Geometry: final body of the model. Coordinates: model frame, mm. Face numbers are marked on the shaded views. A direction names the side the tool comes from. Give positions to 0.01 mm unless a question says otherwise; leave off trailing zeros. Loops run counter-clockwise (first coordinate to the right, second up) from the corner with the lowest first, then second, coordinate; pieces in that order, holes last.
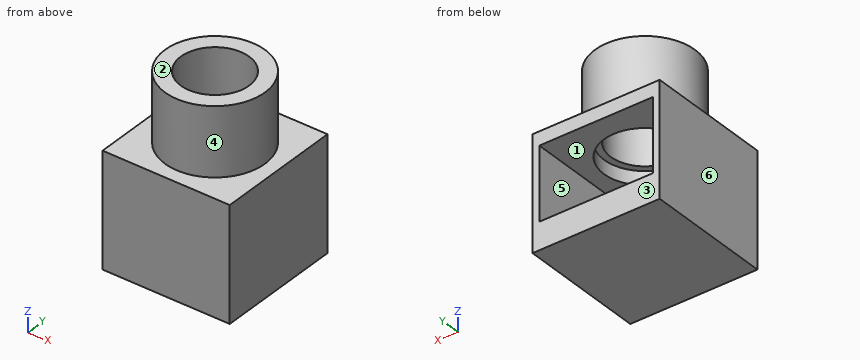
```python
from build123d import *

# Parameters (mm, degrees)
SKETCH1_W           = 7.112
SKETCH1_H           = 6.35
BOSS_EXTRUDE1_DEPTH = 7.112
SKETCH2_R           = 2.286
CUT_EXTRUDE1_DEPTH  = 1.27
SKETCH3_W           = 6.35
SKETCH3_H           = 4.064
CUT_EXTRUDE2_DEPTH  = 6.35
SKETCH4_R           = 2.794
BOSS_EXTRUDE2_DEPTH = 3.81
SKETCH6_R           = 1.907980072
CUT_EXTRUDE3_DEPTH  = 3.81


with BuildPart() as part:
    # Sketch1 → Boss-Extrude1 (new body)
    with BuildSketch(Plane(origin=(0, 0, 0), x_dir=(1, 0, 0), z_dir=(0, 1, 0))):
        with Locations((3.556, 3.175)):
            Rectangle(SKETCH1_W, SKETCH1_H)
    extrude(amount=BOSS_EXTRUDE1_DEPTH)

    # Sketch2 → Cut-Extrude1 (cut)
    with BuildSketch(Plane.XY):
        with Locations((3.556, 3.556)):
            Circle(SKETCH2_R)
    extrude(amount=-CUT_EXTRUDE1_DEPTH, mode=Mode.SUBTRACT)

    # Sketch3 → Cut-Extrude2 (cut)
    with BuildSketch(Plane(origin=(0, 7.112, 0), x_dir=(1, 0, 0), z_dir=(0, 1, 0))):
        with Locations((3.556, 2.794)):
            Rectangle(SKETCH3_W, SKETCH3_H)
    extrude(amount=-CUT_EXTRUDE2_DEPTH, mode=Mode.SUBTRACT)

    # Sketch4 → Boss-Extrude2 (add)
    with BuildSketch(Plane.XY):
        with Locations(Location((3.556, 3.556, 0), (0, 0, 180))):
            Circle(SKETCH4_R)
    extrude(amount=BOSS_EXTRUDE2_DEPTH)

    # Sketch6 → Cut-Extrude3 (cut)
    with BuildSketch(Plane.XY.offset(3.81)):
        with Locations((3.556, 3.556)):
            Circle(SKETCH6_R)
    extrude(amount=-CUT_EXTRUDE3_DEPTH, mode=Mode.SUBTRACT)


solid = part.part
```
Q1. Section query B-B, the plane y = 3. Return loops of the section in (x, z), and give its area (3 significant figures).
Q2. Section query D-D, the plane y = 1.5. Return loops of the section in (x, z), and give its area (3 significant figures).
Q3. Pin query (flat end, axial travel): pin 1 Ø1.2 at (y, z) = (4, -3) entering from -X; pin 2 Ø2 at (x, z) = (3.5, -3) entering from +Y; pin 3 Ø1.9 at (x, y) = (3, 4) entering from +Z. Return the tip coordinate at first contact, or that it passes through.
Q4. Reachability of the marked faces 4, 5 and 6 from +Z, -Z, +X, -X, +Y, -Y: full face, straight path, thin tool, end or side. Return the list, or none.
Q5. Section query C-C, the plane z = -1. Return loops of the section in (x, y), and give its area (3 significant figures).
Q6. Section query A-A, the plane x = 4. Return loops of the section in (y, z), and give its area (3 significant figures).
Q7. Material intervals for probe 1 along X at (y, z) = (3.5, -4.5); probe 2 along Z at (x, y) = (6.25, 3.25); probe 3 along Z at (x, y) = (6, 5.5), sorted ascending.
Q8. Mould query, pull axis Z, two halves, no side actions, for the marked faces 1, 2 and 3. Classes: +Z half, -Z half, draft (parallel to the pull), parting line (faces both ways), or undercut.
Resolved:
1. outline: (0, -6.35) - (7.11, -6.35) - (7.11, 0) - (6.29, 0) - (6.29, 3.81) - (5.38, 3.81) - (5.38, 0) - (5.77, 0) - (5.77, -0.76) - (6.73, -0.76) - (6.73, -4.83) - (0.38, -4.83) - (0.38, -0.76) - (1.34, -0.76) - (1.34, 0) - (1.73, 0) - (1.73, 3.81) - (0.82, 3.81) - (0.82, 0) - (0, 0) - close
1. area: 22.9 mm2
2. outline: (0, -6.35) - (7.11, -6.35) - (7.11, 0) - (5.45, 0) - (5.45, 3.81) - (1.66, 3.81) - (1.66, 0) - (0, 0) - close; hole (0.38, -4.83) - (6.73, -4.83) - (6.73, -0.76) - (4.56, -0.76) - (4.56, 0) - (2.56, 0) - (2.56, -0.76) - (0.38, -0.76) - close
2. area: 32.2 mm2
3. pin 1: stops at x = 0
3. pin 2: stops at y = 0.76
3. pin 3: stops at z = -4.83
4. face 4: +Z
4. face 5: +Y
4. face 6: +Z, -Z, -X, +Y, -Y
5. outline: (0, 0) - (7.11, 0) - (7.11, 7.11) - (6.73, 7.11) - (6.73, 0.76) - (0.38, 0.76) - (0.38, 7.11) - (0, 7.11) - close
5. area: 10.3 mm2
6. outline: (0, -6.35) - (7.11, -6.35) - (7.11, -4.83) - (0.76, -4.83) - (0.76, -0.76) - (1.31, -0.76) - (1.31, 0) - (1.7, 0) - (1.7, 3.81) - (0.8, 3.81) - (0.8, 0) - (0, 0) - close; (5.41, 0) - (5.8, 0) - (5.8, -0.76) - (7.11, -0.76) - (7.11, 0) - (6.31, 0) - (6.31, 3.81) - (5.41, 3.81) - close
6. area: 22.8 mm2
7. probe 1: x = 0 to 0.38, 6.73 to 7.11
7. probe 2: z = -6.35 to -4.83, -0.76 to 3.81
7. probe 3: z = -6.35 to -4.83, -0.76 to 0
8. face 1: undercut
8. face 2: +Z half
8. face 3: draft
